Geometry: final body of the model. Coordinates: model frame, mm. Coordinates: 2 decimals unless noted, no trailing zeros. Order: outer loops, then holes, each group sorted by start corner. A loop starts at its lowest first (then second) coordinate and runs counter-clockwise, first axis right, second up. Notation, with made-up numbers: M 37.25,57.5 L 51.25,57.5 A11 ccw 51.25,72.5 Z; hole C 72,-8 d11. An arc over 180 degrees is marked long. Use CSV: the item, a comma, the result in double quotes. Start each with the question number.
Q1. Section query B-B, the plane z = 8.75. Output: boundary loops of the cut face in (x, y), and give its area (3 significant figures).
Q2. First-contact query: P1, Ø0.5, axis at x = -2.5, z = 22.5, coming from the +Y side; P2, Ø1.1, axis at y = -1, z = 24, coming from the -X side; P3, Ø4, axis at x = -3, z = 10, coming from the +Y side. Flat tips, straight axial feed; report the tip coordinate or a pass-through.
Q3. Section query D-D, the plane y = 1.75. Output: boundary loops of the cut face in (x, z), and give its area (3 significant figures).
Q4. Section query A-A, the plane x = -2.5. Output: boundary loops of the cut face in (y, z).
Q5. Section query C-C, the plane y = -3. Output: boundary loops of the cut face in (x, z), and give its area (3 significant figures).
Q6. Ray query, probe 1 along Z at (x, y) = (0.75, 0.5); probe 2 along Y at (x, z) = (3.25, 7); probe 3 along X at (y, z) = (-4.5, 20.25). Return the intervals inside material, ascending.
from build123d import *

# Parameters (mm, degrees)
F0_R     = 5.08
F1_DEPTH = 25.4
F3_DEPTH = 5.08


with BuildPart() as f1:
    # F0 (on Top) → F1 (new body)
    with BuildSketch(Plane.XY):
        Circle(F0_R)
    extrude(amount=F1_DEPTH)

    # F2 (on face) → F3 (cut)
    with BuildSketch(Plane.XY.offset(25.4)):
        Polygon((-3.493968, 1.360344), (-3.493968, -1.511888), (-2.840127, -1.511888), (-2.840127, 0), (-1.933453, 0), (-1.933453, 0.426284), (-2.816775, 0.426284), (-2.816775, 0.776557), (-1.933453, 0.776557), (-1.933453, 1.360344), align=None)
        with BuildLine():
            Line((0, 1.360344), (-1.042063, 1.360344))
            Line((-1.042063, 1.360344), (-1.042063, -1.511888))
            Line((-1.042063, -1.511888), (-0.318167, -1.511888))
            Line((-0.318167, -1.511888), (-0.318167, -0.484423))
            Line((-0.318167, -0.484423), (0.335674, -1.511888))
            Line((0.335674, -1.511888), (1.036218, -1.511888))
            Line((1.036218, -1.511888), (0.330819, -0.403403))
            ThreePointArc((0.330819, -0.403403), (0.897252, 0.615739), (0, 1.360344))
        make_face()
    extrude(amount=-F3_DEPTH, mode=Mode.SUBTRACT)


solid = f1.part
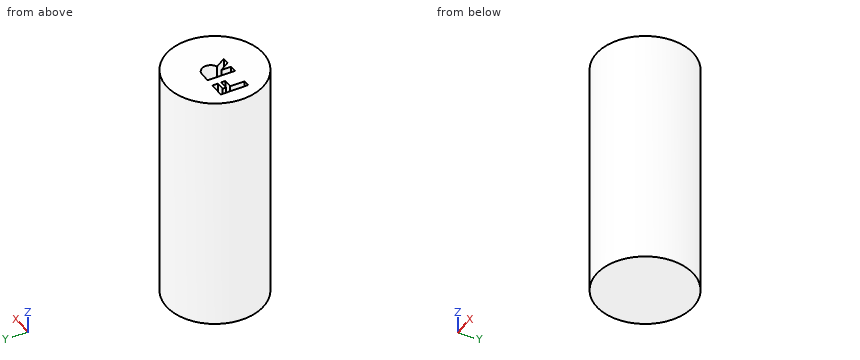
Responses:
1,outline,"C 0,0 d10.16"
1,area,"81.1 mm²"
2,P1,"stops at y = 4.55"
2,P2,"stops at x = -5.06"
2,P3,"stops at y = 4.98"
3,outline,"M -4.77,0 L 4.77,0 L 4.77,25.4 L -4.77,25.4 Z"
3,area,"242 mm²"
4,outline,"M -4.42,0 L 4.42,0 L 4.42,25.4 L 1.36,25.4 L 1.36,20.32 L 0.78,20.32 L 0.78,25.4 L 0.43,25.4 L 0.43,20.32 L 0,20.32 L 0,25.4 L -4.42,25.4 Z"
5,outline,"M -4.1,0 L 4.1,0 L 4.1,25.4 L -4.1,25.4 Z"
5,area,"208 mm²"
6,probe 1,"z = 0 to 20.32"
6,probe 2,"y = -3.9 to 3.9"
6,probe 3,"x = -2.36 to 2.36"
